```python
from build123d import *

# Parameters (mm, degrees)
SKETCH_1_R      = 1.5
EXTRUDE_1_DEPTH = 3


with BuildPart() as part:
    # 草图1 → 凸台-拉伸1 (new body)
    with BuildSketch(Plane.XY):
        with BuildLine():
            ThreePointArc((3.16227766, 1.5), (-3.5, 0), (3.16227766, -1.5))
            Line((3.16227766, -1.5), (3.16227766, 1.5))
        make_face()
        Circle(SKETCH_1_R, mode=Mode.SUBTRACT)
        with BuildLine():
            ThreePointArc((3.5, 0), (3.414525722, -0.768774411), (3.16227766, -1.5))
            Line((3.16227766, -1.5), (27.83772234, -1.5))
            ThreePointArc((27.83772234, -1.5), (27.5, 0), (27.83772234, 1.5))
            Line((27.83772234, 1.5), (3.16227766, 1.5))
            ThreePointArc((3.16227766, 1.5), (3.414525722, 0.768774411), (3.5, 0))
        make_face()
        with BuildLine():
            Line((27.83772234, 1.5), (27.83772234, -1.5))
            ThreePointArc((27.83772234, -1.5), (31.768774411, -3.414525722), (34.5, 0))
            ThreePointArc((34.5, 0), (31.768774411, 3.414525722), (27.83772234, 1.5))
        make_face()
        with Locations((31, 0)):
            Circle(SKETCH_1_R, mode=Mode.SUBTRACT)
        with BuildLine():
            Line((3.16227766, 1.5), (3.16227766, -1.5))
            ThreePointArc((3.16227766, -1.5), (3.414525722, -0.768774411), (3.5, 0))
            ThreePointArc((3.5, 0), (3.414525722, 0.768774411), (3.16227766, 1.5))
        make_face()
        with BuildLine():
            ThreePointArc((27.83772234, 1.5), (27.5, 0), (27.83772234, -1.5))
            Line((27.83772234, -1.5), (27.83772234, 1.5))
        make_face()
    extrude(amount=EXTRUDE_1_DEPTH)


solid = part.part
```
Can you work these out from the model? Positions are in its coordinate system, mm. A direction names the side the tool comes from. Coordinates: 2 decimals unless noted, no trailing zeros. Write each loop counter-clockwise with the first axis right and the second up, starting at its lowest first coordinate (ties: lowest second). Pieces come first, ordered by that corner, then holes. Notation, with made-up numbers: M 14.25,78.5 L 42.25,78.5 A17 ccw 42.25,97.5 Z; hole C -17.75,23 d8. An arc over 180 degrees is marked long. Answer as CSV lines item,"result".
Item 1: Imagine slicing it at B-B on x = 31. List the corners of the cut face in (y, z) for me.
Geometry results:
outline,"M -3.5,0 L -1.5,0 L -1.5,3 L -3.5,3 Z; M 1.5,0 L 3.5,0 L 3.5,3 L 1.5,3 Z"
Item 2: On a 3-axis mill with a long thin cutter (end or side, diameter ignored), from which of +Z, -Z, +X, -X, +Y, -Y can I reach the whole of each face in a straight line? I mean faces 3 (the flat face through (15, 0, 3)), 4 (the flat face through (15, -1.5, 1)), 5 (the flat face through (16, 1.5, 1)). Say none if no direction works.
Geometry results:
face 3,"+Z, +X, -X, +Y, -Y"
face 4,"+Z, -Z, -Y"
face 5,"+Z, -Z, +Y"
Item 3: Imagine slicing it at D-D on x = 26.5. List the corners of the cut face in (y, z) for me, plus the area to 3 significant figures.
Geometry results:
outline,"M -1.5,0 L 1.5,0 L 1.5,3 L -1.5,3 Z"
area,"9.00 mm2"
Item 4: I'm going to push flat-ended pins straight in: P1, Ø0.9, axis at x = 16.5, z = 1.5, coming from the +Y side; P2, Ø2, axis at x = 23.5, y = 0.5, coming from the -Z side; P3, Ø1.5, axis at x = 20.5, z = 1, coming from the -Y side. Where does each tip first touch, or does it pass through?
Geometry results:
P1,"stops at y = 1.5"
P2,"stops at z = 0"
P3,"stops at y = -1.5"
Item 5: Please list where these lines run through material, in increasing order: line 1 along X through (y, z) = (-1, 1.15); line 2 along X through (y, z) = (1.25, 2.7); line 3 along Y through (x, z) = (0, 0.8).
Geometry results:
line 1,"x = -3.35 to -1.12, 1.12 to 29.88, 32.12 to 34.35"
line 2,"x = -3.27 to -0.83, 0.83 to 30.17, 31.83 to 34.27"
line 3,"y = -3.5 to -1.5, 1.5 to 3.5"
Item 6: We'd pull the mould along X, two halves only. Please class faces 1 (the flat face through (15, 0, 0)), 2 (the cylindrical face through (29.5, 0.07, 1.48)): +X half, -X half, draft (parallel to the pull), parting line (faces both ways), or undercut.
Geometry results:
face 1,"draft"
face 2,"undercut"
Item 7: Imagine slicing it at C-C on y = 3. List the corners of the cut face in (x, z) for me, plus the area to 3 significant figures.
Geometry results:
outline,"M -1.8,0 L 1.8,0 L 1.8,3 L -1.8,3 Z; M 29.2,0 L 32.8,0 L 32.8,3 L 29.2,3 Z"
area,"21.6 mm2"
Item 8: Imagine slicing it at A-A on z = 0.85. List the corners of the cut face in (x, y) for me, plus the area to 3 significant figures.
Geometry results:
outline,"M 3.16,-1.5 L 27.84,-1.5 A3.5 ccw long 27.84,1.5 L 3.16,1.5 A3.5 ccw long Z; hole C 0,0 d3; hole C 31,0 d3"
area,"135 mm2"
